```python
from build123d import *

# Parameters (mm, degrees)
BOSS_EXTRUDE1_DEPTH = 5


with BuildPart() as part:
    # Sketch1 → Boss-Extrude1 (new body)
    with BuildSketch(Plane.XY):
        with BuildLine():
            Line((117.9, 12), (215.7, 12))
            Line((215.7, 12), (215.7, 16))
            ThreePointArc((215.7, 16), (215.992893219, 16.707106781), (216.7, 17))
            Line((216.7, 17), (224.6, 17))
            ThreePointArc((224.6, 17), (225.307106781, 16.707106781), (225.6, 16))
            Line((225.6, 16), (225.6, 1))
            ThreePointArc((225.6, 1), (225.307106781, 0.292893219), (224.6, 0))
            Line((224.6, 0), (1, 0))
            ThreePointArc((1, 0), (0.292893219, 0.292893219), (0, 1))
            Line((0, 1), (0, 16))
            ThreePointArc((0, 16), (0.292893219, 16.707106781), (1, 17))
            Line((1, 17), (9, 17))
            ThreePointArc((9, 17), (9.707106781, 16.707106781), (10, 16))
            Line((10, 16), (10, 12))
            Line((10, 12), (107.8, 12))
            Line((107.8, 12), (107.8, 16))
            ThreePointArc((107.8, 16), (108.092893219, 16.707106781), (108.8, 17))
            Line((108.8, 17), (116.9, 17))
            ThreePointArc((116.9, 17), (117.607106781, 16.707106781), (117.9, 16))
            Line((117.9, 16), (117.9, 12))
        make_face()
    extrude(amount=BOSS_EXTRUDE1_DEPTH)


solid = part.part
```
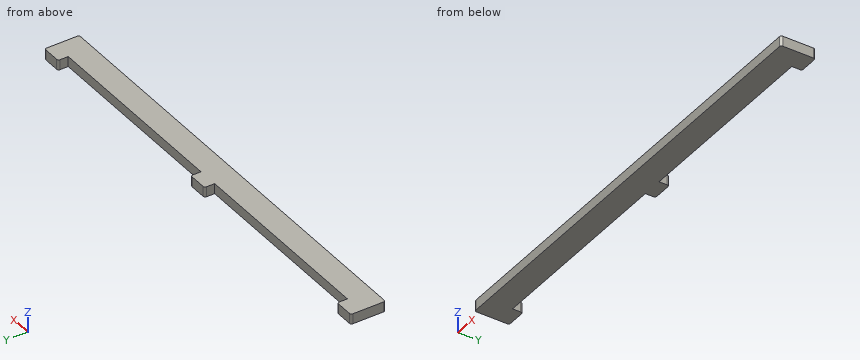
CAD build for the part. Positions are in the model's coordinates, mm. Round coordinates to 2 decimals unless told otherwise and drop trailing zeros. Order: outer loops, then holes, each group sorted by start corner. A loop starts at its lowest first (then second) coordinate and runs counter-clockwise, first axis right, second up. Notation, with made-up numbers: (50, 76.5) -> (95, 76.5) arc R16 ccw to (95, 94.5) -> close; hole circle Ø11 at (37, -7.5). An arc over 180 degrees is marked (long way). One line per question, with ' | ' between items.
Q1. Slice it at B-B (z = 2.4). Write the cut outline in (x, y), then the cut area to 3 significant figures.
Completed:
outline: (0, 1) arc R1 ccw to (1, 0) -> (224.6, 0) arc R1 ccw to (225.6, 1) -> (225.6, 16) arc R1 ccw to (224.6, 17) -> (216.7, 17) arc R1 ccw to (215.7, 16) -> (215.7, 12) -> (117.9, 12) -> (117.9, 16) arc R1 ccw to (116.9, 17) -> (108.8, 17) arc R1 ccw to (107.8, 16) -> (107.8, 12) -> (10, 12) -> (10, 16) arc R1 ccw to (9, 17) -> (1, 17) arc R1 ccw to (0, 16) -> close | area: 2,860 mm^2
Q2. Probe probe 1 along X at (y, z) = (12.25, 2.75); probe 2 along Y at (x, z) = (143, 1.6). List the from-to ranges inside material, lowest first.
Completed:
probe 1: x = 0 to 10, 107.8 to 117.9, 215.7 to 225.6 | probe 2: y = 0 to 12
Q3. Drop a flat-ended pin along its axis: pin 1 (1.5 mm diameter, centred on x = 61, z = 2, fed in from +Y). Give the stop position or say it passes through.
Completed:
pin 1: stops at y = 12
Q4. Slice it at C-C (x = 169.5). Write the cut outline in (y, z), then the cut area to 3 significant figures.
Completed:
outline: (0, 0) -> (12, 0) -> (12, 5) -> (0, 5) -> close | area: 60.0 mm^2
Q5. Slice it at A-A (y = 14). Write the cut outline in (x, z).
Completed:
outline: (0, 0) -> (10, 0) -> (10, 5) -> (0, 5) -> close; (107.8, 0) -> (117.9, 0) -> (117.9, 5) -> (107.8, 5) -> close; (215.7, 0) -> (225.6, 0) -> (225.6, 5) -> (215.7, 5) -> close
